from build123d import *

# Parameters (mm, degrees)
SKETCH_1_W                       = 25
SKETCH_1_H                       = 25
EXTRUDE_1_DEPTH                  = 64
CUT_EXTRUDE_1_DEPTH              = 100
CUT_EXTRUDE_4_DEPTH              = 64
SKETCH_3_W                       = 38
SKETCH_3_H                       = 25
EXTRUDE_2_DEPTH                  = 3
SKETCH_4_R                       = 1
CUT_EXTRUDE_2_DEPTH              = 3
PATTERN_LINEAR_1_COUNT           = 2
PATTERN_LINEAR_1_PITCH           = 32
PATTERN_LINEAR_2_COUNT           = 2
PATTERN_LINEAR_2_PITCH           = 16
PATTERN_LINEAR_2_COPY_1_SKETCH_R = 1
PATTERN_LINEAR_2_COPY_1_DEPTH    = 3
SKETCH_6_W                       = 9.9
SKETCH_6_H                       = 5.8
EXTRUDE_3_DEPTH                  = 3
SKETCH_7_W                       = 34
SKETCH_7_H                       = 25
EXTRUDE_4_DEPTH                  = 3
SKETCH_8_R                       = 1
CUT_EXTRUDE_3_DEPTH              = 3
PATTERN_CIRCULAR_1_COUNT         = 4


with BuildPart() as part:
    # 草图1 → 凸台-拉伸1 (new body)
    with BuildSketch(Plane.XY):
        Rectangle(SKETCH_1_W, SKETCH_1_H)
    extrude(amount=EXTRUDE_1_DEPTH)

    # 草图2 → 切除-拉伸1 (cut)
    with BuildSketch(Plane(origin=(0, 0, 0), x_dir=(-1, 0, 0), z_dir=(0, 0, -1))):
        Polygon((-4.5, 1.5), (-12.5, 9.5), (-12.5, -9.5), (-4.5, -1.5), align=None)
    cut_extrude_1 = extrude(amount=-CUT_EXTRUDE_1_DEPTH, mode=Mode.SUBTRACT)

    # 镜向1: 切除-拉伸1 across plane
    add(cut_extrude_1.mirror(Plane(origin=(0, 0, 0), x_dir=(0, 0, 1), z_dir=(1, 0, 0))), mode=Mode.SUBTRACT)

    # 草图9 → 切除-拉伸4 (cut)
    with BuildSketch(Plane(origin=(0, 0, 0), x_dir=(-1, 0, 0), z_dir=(0, 0, -1))):
        Polygon((-8, 12.5), (0, 4.5), (8, 12.5), align=None)
    cut_extrude_4 = extrude(amount=-CUT_EXTRUDE_4_DEPTH, mode=Mode.SUBTRACT)

    # 镜向2: 切除-拉伸4 across plane
    add(cut_extrude_4.mirror(Plane.ZX), mode=Mode.SUBTRACT)

    # 草图3 → 凸台-拉伸2 (add)
    with BuildSketch(Plane(origin=(0, 0, 0), x_dir=(-1, 0, 0), z_dir=(0, 0, -1))):
        Rectangle(SKETCH_3_W, SKETCH_3_H)
    extrude(amount=EXTRUDE_2_DEPTH)

    # 草图4 → 切除-拉伸2 (cut)
    with BuildSketch(Plane(origin=(0, 0, -3), x_dir=(-1, 0, 0), z_dir=(0, 0, -1))):
        with Locations((-16, 8)):
            Circle(SKETCH_4_R)
    cut_extrude_2 = extrude(amount=-CUT_EXTRUDE_2_DEPTH, mode=Mode.SUBTRACT)

    # 阵列(线性)1: 切除-拉伸2 ×2
    with Locations(*[(-i * PATTERN_LINEAR_1_PITCH, 0, 0) for i in range(1, PATTERN_LINEAR_1_COUNT)]):
        add(cut_extrude_2, mode=Mode.SUBTRACT)

    # 阵列(线性)2: 切除-拉伸2 ×2
    with Locations(*[(0, -i * PATTERN_LINEAR_2_PITCH, 0) for i in range(1, PATTERN_LINEAR_2_COUNT)]):
        add(cut_extrude_2, mode=Mode.SUBTRACT)

    # 阵列(线性)2 copy 1 sketch → 阵列(线性)2 copy 1 (cut)
    with BuildSketch(Plane(origin=(-32, -16, -3), x_dir=(-1, 0, 0), z_dir=(0, 0, -1))):
        with Locations((-16, 8)):
            Circle(PATTERN_LINEAR_2_COPY_1_SKETCH_R)
    extrude(amount=-PATTERN_LINEAR_2_COPY_1_DEPTH, mode=Mode.SUBTRACT)

    # 草图6 → 凸台-拉伸3 (add)
    with BuildSketch(Plane(origin=(0, 0, -3), x_dir=(-1, 0, 0), z_dir=(0, 0, -1))):
        Rectangle(SKETCH_6_W, SKETCH_6_H)
    extrude(amount=EXTRUDE_3_DEPTH)

    # 草图7 → 凸台-拉伸4 (add)
    with BuildSketch(Plane.XY.offset(64)):
        Rectangle(SKETCH_7_W, SKETCH_7_H)
    extrude(amount=EXTRUDE_4_DEPTH)

    # 草图8 → 切除-拉伸3 (cut)
    with BuildSketch(Plane.XY.offset(67)):
        with Locations((0, 8)):
            Circle(SKETCH_8_R)
    cut_extrude_3 = extrude(amount=-CUT_EXTRUDE_3_DEPTH, mode=Mode.SUBTRACT)

    # 阵列(圆周)1: 切除-拉伸3 ×4 about axis
    pattern_circular_1_axis = Axis((0, 0, 0), (0, 0, 1))
    for i in range(1, PATTERN_CIRCULAR_1_COUNT):
        add(cut_extrude_3.rotate(pattern_circular_1_axis, i * 360 / PATTERN_CIRCULAR_1_COUNT), mode=Mode.SUBTRACT)


solid = part.part
Build history of the part. All positions in model axes, mm. A direction names the side the tool comes from. Round coordinates to 2 decimals unless told otherwise and drop trailing zeros. Loops run counter-clockwise (first coordinate to the right, second up) from the corner with the lowest first, then second, coordinate; pieces in that order, holes last. Notation, with made-up numbers: (-28.75, -31) -> (26.25, -31) arc R6 cw to (26.25, -22) -> close; hole circle Ø2 at (-25, -1.75). An arc over 180 degrees is marked (long way). Use CSV: the item, a comma, the result in double quotes. Start each with the question number.
Q1. Saw through at D-D on x = 6. Give the cut face in (y, z), and give its area (3 significant figures).
Q2. Flat gauge pins, fed straight in: pin 1 Ø1 at (x, z) = (3, 24.5) entering from -Y; pin 2 Ø9 at (x, y) = (-3.5, 8) entering from -Z; pin 3 Ø2.5 at (y, z) = (-11, 45.5) entering from +X. Where does each tip first touch, or does it go through?
Q3. Mould opens along Z. For faces 1 (the face through (15, -8, -2)), 2 (the face through (-3.9, 8.4, 31.6)), 3 (the face through (0, 0, -6)) say: +Z half, -Z half, draft (parallel to the pull), parting line (faces both ways), or undercut.
Q4. Saw through at A-A on x = 16. Give the cut face in (y, z), and give its area (3 significant figures).
Q5. Saw through at B-B on y = 8. Give the cut face in (x, z).
Q6. Which spindle directions (+Z, -Z, +X, -X, +Y, -Y) get a long thin tool onto all of the face, cutting with end or side? Do faces 4 (the face through (4.95, 0, -4)), 5 (the face through (4.1, -8.6, 31.6)), 6 (the face through (0, 9, 0)). Say none if no direction does.
Q7. Saw through at C-C on z = 38.5. Give the cut face in (x, y), and give its area (3 significant figures).
Q8. Drill centre lines: L1, parallel to Y at x = 0, z = 65.1; L2, parallel to Y at x = 12, z = 41; L3, parallel to Z at x = 15, y = 2.5. Where is each one in solid material? Low to high.
Solutions:
1,outline,"(-12.5, -3) -> (12.5, -3) -> (12.5, 0) -> (10.5, 0) -> (10.5, 64) -> (12.5, 64) -> (12.5, 67) -> (-12.5, 67) -> (-12.5, 64) -> (-10.5, 64) -> (-10.5, 0) -> (-12.5, 0) -> close; hole (-3, 0) -> (3, 0) -> (3, 64) -> (-3, 64) -> close"
1,area,"1,110 mm^2"
2,pin 1,"stops at y = -8"
2,pin 2,"stops at z = -3"
2,pin 3,"stops at x = 12.5"
3,face 1,"draft"
3,face 2,"undercut"
3,face 3,"-Z half"
4,outline,"(-12.5, -3) -> (-9, -3) -> (-9, 0) -> (-12.5, 0) -> close; (-12.5, 64) -> (12.5, 64) -> (12.5, 67) -> (-12.5, 67) -> close; (-7, -3) -> (7, -3) -> (7, 0) -> (-7, 0) -> close; (9, -3) -> (12.5, -3) -> (12.5, 0) -> (9, 0) -> close"
4,area,"138 mm^2"
5,outline,"(-19, -3) -> (-17, -3) -> (-17, 0) -> (-19, 0) -> close; (-17, 64) -> (-11, 64) -> (-11, 0) -> (-15, 0) -> (-15, -3) -> (15, -3) -> (15, 0) -> (11, 0) -> (11, 64) -> (17, 64) -> (17, 67) -> (1, 67) -> (1, 64) -> (3.5, 64) -> (3.5, 0) -> (-3.5, 0) -> (-3.5, 64) -> (-1, 64) -> (-1, 67) -> (-17, 67) -> close; (17, -3) -> (19, -3) -> (19, 0) -> (17, 0) -> close"
6,face 4,"-Z, +X, +Y, -Y"
6,face 5,"-Y"
6,face 6,"+Y"
7,outline,"(-12.5, -12.5) -> (-8, -12.5) -> (0, -4.5) -> (8, -12.5) -> (12.5, -12.5) -> (12.5, -9.5) -> (4.5, -1.5) -> (4.5, 1.5) -> (12.5, 9.5) -> (12.5, 12.5) -> (8, 12.5) -> (0, 4.5) -> (-8, 12.5) -> (-12.5, 12.5) -> (-12.5, 9.5) -> (-4.5, 1.5) -> (-4.5, -1.5) -> (-12.5, -9.5) -> close"
7,area,"321 mm^2"
8,L1,"y = -12.5 to -9, -7 to 7, 9 to 12.5"
8,L2,"y = -12.5 to -9, 9 to 12.5"
8,L3,"z = -3 to 0, 64 to 67"
